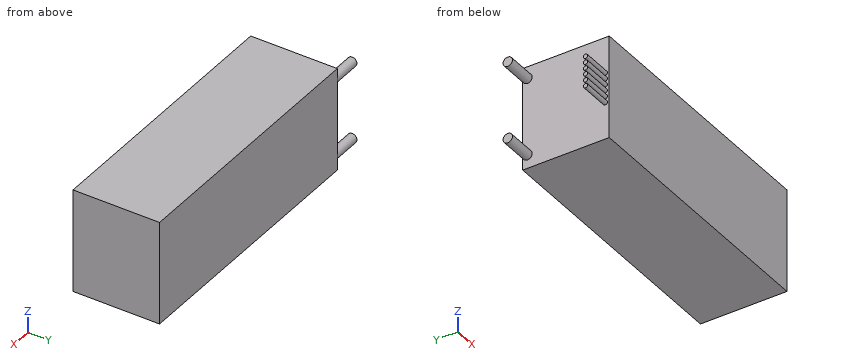
from build123d import *

# Parameters (mm, degrees)
SKETCH_1_W      = 135
SKETCH_1_H      = 51.7
EXTRUDE_1_DEPTH = 43.34
SKETCH_2_R      = 1.086280141
SKETCH_2_R_2    = 2.372753638
SKETCH_2_R_3    = 2.361962499
EXTRUDE_2_DEPTH = 15


with BuildPart() as part:
    # 草图1 → 凸台-拉伸1 (new body)
    with BuildSketch(Plane(origin=(0, 0, 0), x_dir=(1, 0, 0), z_dir=(0, 1, 0))):
        with Locations((67.5, 25.85)):
            Rectangle(SKETCH_1_W, SKETCH_1_H)
    extrude(amount=EXTRUDE_1_DEPTH)

    # 草图2 → 凸台-拉伸2 (add)
    with BuildSketch(Plane.ZY):
        with Locations((-33.248816044, 1.972664588)):
            Circle(SKETCH_2_R)
        with Locations((-45.037596274, 40.939762419)):
            Circle(SKETCH_2_R_2)
        with Locations((-6.119823883, 40.939762419)):
            Circle(SKETCH_2_R_3)
        with Locations((-30.248816044, 1.972664588)):
            Circle(SKETCH_2_R)
        with Locations((-27.248816044, 1.972664588)):
            Circle(SKETCH_2_R)
        with Locations((-24.248816044, 1.972664588)):
            Circle(SKETCH_2_R)
        with Locations((-21.248816044, 1.972664588)):
            Circle(SKETCH_2_R)
        with Locations((-18.248816044, 1.972664588)):
            Circle(SKETCH_2_R)
    extrude(amount=EXTRUDE_2_DEPTH)


solid = part.part
Part model, mm, in its own coordinate system. Give positions to 0.01 mm unless a question says otherwise; leave off trailing zeros. Loops run counter-clockwise (first coordinate to the right, second up) from the corner with the lowest first, then second, coordinate; pieces in that order, holes last.
(1) Band-saw the part on B-B (y = 33). Write the cut outline in (x, z), and give its area (3 significant figures).
Return value:
outline: (0, -51.7) - (135, -51.7) - (135, 0) - (0, 0) - close
area: 6,980 mm2
(2) Pin check, flat tip, straight feed: pin 1 (12 mm diameter, centred on y = 22.5, z = -34, fed in from -X). Stop position of the tip, or through.
Return value:
pin 1: stops at x = 0
(3) Drill centre lines: line 1 along X through (y, z) = (35, -12); line 2 along Y through (x, z) = (-7, -18.5). Where is each one in solid material? Low to high.
Return value:
line 1: x = 0 to 135
line 2: y = 0.92 to 3.03
(4) Band-saw the part on A-A (z = -44). Write the cut outline in (x, y), and give its area (3 significant figures).
Return value:
outline: (-15, 38.81) - (0, 38.81) - (0, 0) - (135, 0) - (135, 43.34) - (0, 43.34) - (0, 43.07) - (-15, 43.07) - close
area: 5,910 mm2
